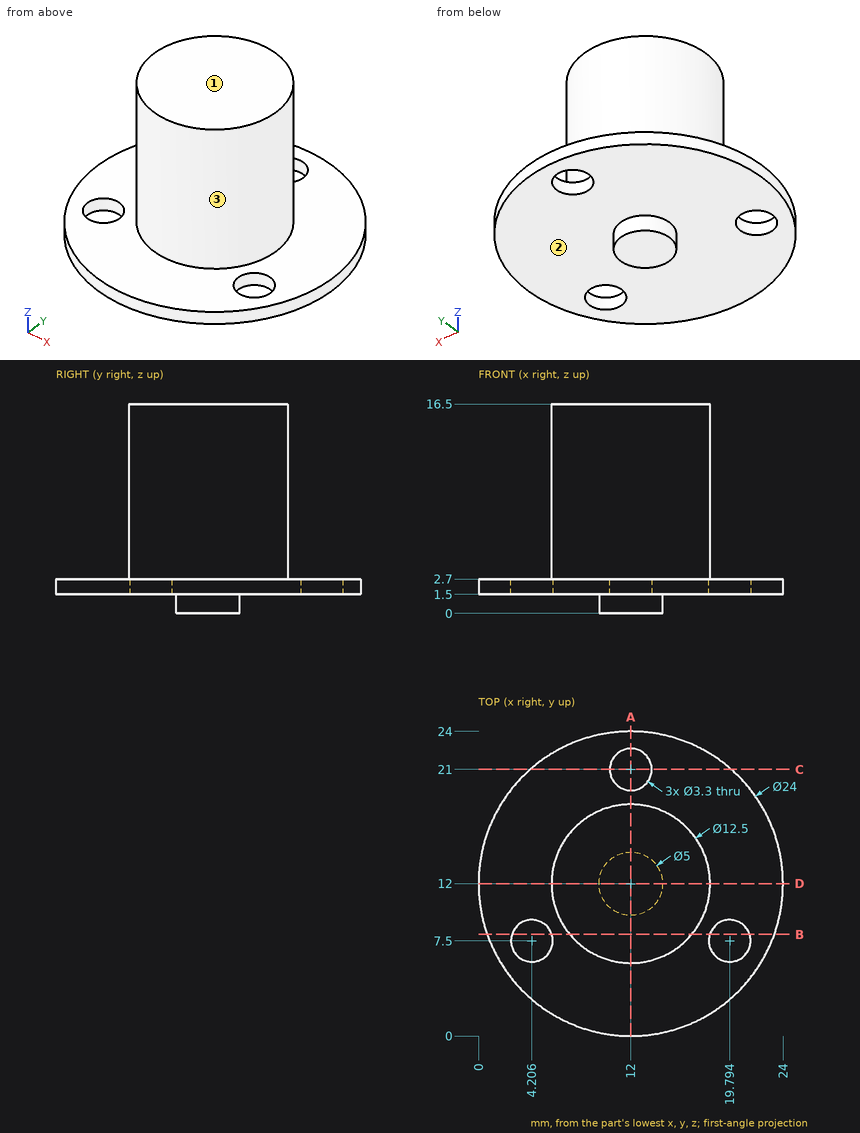
Part print with two shaded views. Sizes in mm from the minimum x, y, z corner. A direction names the side the tool comes from. Round coordinates to 2 decimals unless told otherwise and drop trailing zeros. Loops run counter-clockwise (first coordinate to the right, second up) from the corner with the lowest first, then second, coordinate; pieces in that order, holes last.
Item 1: Which spindle directions (+Z, -Z, +X, -X, +Y, -Y) get a long thin tool onto all of the face, cutting with end or side? Do the marked faces 1, 2 and 3. Say none if no direction does.
Item 2: Pin check, flat tips, straight feed: P1, Ø4.5, axis at x = 19.79, y = 7.5, coming from the +Z side; P2, Ø5, axis at y = 13.5, z = 5.5, coming from the -X side; P3, Ø2, axis at x = 4.21, y = 7.5, coming from the +Z side; P4, Ø12, axis at x = 13, y = 6.5, coming from the -Z side. Stop position of each tip, or through.
Item 3: Drill centre lines: line 1 along X through (y, z) = (6.25, 2.25); line 2 along X through (y, z) = (11.75, 15.5) (1 decimal); line 3 along Z through (x, y) = (17.25, 13). Where is each one in solid material? Low to high.
Item 4: Saw through at D-D (y = 12). List the corners of the cut face in (x, z), then the cut area to 3 significant figures.
Item 5: Saw through at A-A (x = 12). List the corners of the cut face in (y, z), then the cut area to 3 significant figures.
Item 6: Saw through at B-B (y = 8). List the corners of the cut face in (x, z), then the cut area to 3 significant figures.
Item 7: Saw through at C-C (y = 21). List the corners of the cut face in (x, z).
Worked answers:
1. face 1: +Z, +X, -X, +Y, -Y
1. face 2: -Z
1. face 3: +Z
2. P1: stops at z = 2.7
2. P2: stops at x = 5.75
2. P3: passes through
2. P4: stops at z = 0
3. line 1: x = 1.47 to 3.13, 5.28 to 18.72, 20.87 to 22.53
3. line 2: x = 5.8 to 18.2
3. line 3: z = 1.5 to 16.5
4. outline: (0, 1.5) - (9.5, 1.5) - (9.5, 0) - (14.5, 0) - (14.5, 1.5) - (24, 1.5) - (24, 2.7) - (18.25, 2.7) - (18.25, 16.5) - (5.75, 16.5) - (5.75, 2.7) - (0, 2.7) - close
4. area: 209 mm2
5. outline: (0, 1.5) - (9.5, 1.5) - (9.5, 0) - (14.5, 0) - (14.5, 1.5) - (19.35, 1.5) - (19.35, 2.7) - (18.25, 2.7) - (18.25, 16.5) - (5.75, 16.5) - (5.75, 2.7) - (0, 2.7) - close; (22.65, 1.5) - (24, 1.5) - (24, 2.7) - (22.65, 2.7) - close
5. area: 205 mm2
6. outline: (0.69, 1.5) - (2.63, 1.5) - (2.63, 2.7) - (0.69, 2.7) - close; (5.78, 1.5) - (18.22, 1.5) - (18.22, 2.7) - (16.8, 2.7) - (16.8, 16.5) - (7.2, 16.5) - (7.2, 2.7) - (5.78, 2.7) - close; (21.37, 1.5) - (23.31, 1.5) - (23.31, 2.7) - (21.37, 2.7) - close
6. area: 152 mm2
7. outline: (4.06, 1.5) - (10.35, 1.5) - (10.35, 2.7) - (4.06, 2.7) - close; (13.65, 1.5) - (19.94, 1.5) - (19.94, 2.7) - (13.65, 2.7) - close
